Autodesk Inventor part; units mm, degrees
ref_plane "YZ Plane" through (0, 0, 0) normal (1, 0, 0) x (0, 1, 0)
ref_plane "XZ Plane" through (0, 0, 0) normal (0, 1, 0) x (-1, 0, 0)
ref_plane "XY Plane" through (0, 0, 0) normal (0, 0, 1) x (1, 0, 0)
sketch "スケッチ1" plane through (0, 0, 0) normal (0, 0, 1) x (1, 0, 0)
  circle A0 centre (12.3759, 55.251) radius 1.5
  circle A1 centre (22.7017, 77.6457) radius 1.5
  circle A2 centre (20.6799, 65) radius 1.5
  circle A3 centre (22.7017, 77.6457) radius 4.5
  circle A4 centre (20.6799, 65) radius 4.5
  circle A5 centre (12.3759, 55.251) radius 4.5
  line L0 (8.9502, 58.1689) -> (17.2542, 67.918)
  line L1 (18.2581, 78.3561) -> (16.2364, 65.7104)
  line L2 (27.1453, 76.9352) -> (25.1235, 64.2896)
  line L3 (15.8017, 52.333) -> (24.1057, 62.082)
  point P0 (0, 0)
  point P1 (0, 0)
  point P2 (16.4357, 66.957)
  dimension "d0" = 3
  dimension "d1" = 3
  dimension "d2" = 3
extrude "押し出し1" add sketch "スケッチ1" along normal blind 3
properties part number "段ばね抑え2" material "アセタール樹脂、白"
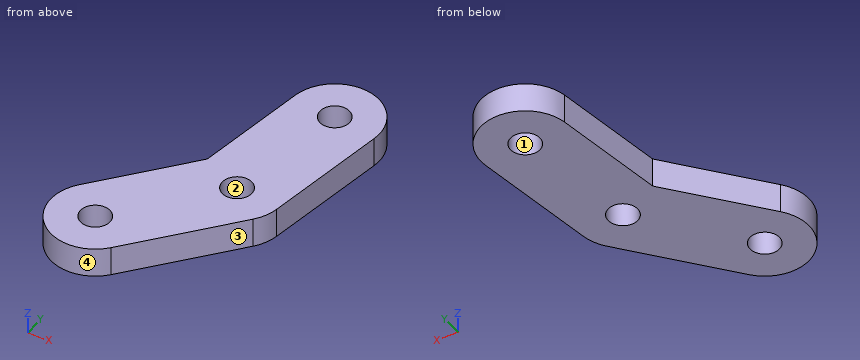
Here's how the part is built. I have some questions about the finished solid (model axes, mm). Face numbers are marked on the shaded views. Round coordinates to 2 decimals unless told otherwise and drop trailing zeros. Order: outer loops, then holes, each group sorted by start corner. A loop starts at its lowest first (then second) coordinate and runs counter-clockwise, first axis right, second up. Notation, with made-up numbers: (19, -32) -> (25, -32) arc R19 ccw to (25, -1) -> close; hole circle Ø1 at (25.5, -18). An arc over 180 degrees is marked (long way). Use CSV: the item, a comma, the result in double quotes.
1. I want a section at A-A on x = 12. List the corners of the cut face in (y, z) for me, and give its area (3 significant figures).
Recorded:
outline,"(50.77, 0) -> (53.8, 0) -> (53.8, 3) -> (50.77, 3) -> close; (56.7, 0) -> (61.75, 0) -> (61.75, 3) -> (56.7, 3) -> close"
area,"24.2 mm2"
2. Thinking about a two-plate mould opening in Y: for the marked faces 1, 2, 3 and 4, which applies, pulls with the +Y half, pulls with the -Y half, needs draft (parallel to the pull), parting line crosses it, or undercut?
Recorded:
face 1,"undercut"
face 2,"undercut"
face 3,"pulls with the -Y half"
face 4,"parting line crosses it"
3. I need wall thicknesses on line 1 along Y through (x, z) = (21.5, 0.85); line 2 along X through (y, z) = (79, 0.65); line 3 along Y through (x, z) = (11.75, 1.6). Which ranges of each line are inside material? Lowest first, please.
Recorded:
line 1,"y = 59.02 to 63.74, 66.26 to 76.75, 78.54 to 81.98"
line 2,"x = 18.41 to 22.06, 23.35 to 26.99"
line 3,"y = 50.79 to 53.89, 56.61 to 61.46"
4. I want a section at D-D on y = 79.5. List the corners of the cut face in (x, z) for me.
Recorded:
outline,"(18.6, 0) -> (26.8, 0) -> (26.8, 3) -> (18.6, 3) -> close"
5. I want a section at B-B on y = 56. List the corners of the cut face in (x, z) for me, and give its area (3 significant figures).
Recorded:
outline,"(7.94, 0) -> (11.08, 0) -> (11.08, 3) -> (7.94, 3) -> close; (13.68, 0) -> (18.93, 0) -> (18.93, 3) -> (13.68, 3) -> close"
area,"25.2 mm2"
6. I'm going to push a flat-ended pin straight in: P1, Ø1, axis at x = 16.5, z = 2, coming from the -Y side. Where does the tip first touch, or does it pass through?
Recorded:
P1,"stops at y = 52.57"
7. I want a section at C-C on z = 1.7. List the corners of the cut face in (x, y) for me, and give its area (3 significant figures).
Recorded:
outline,"(8.95, 58.17) arc R4.5 ccw to (15.8, 52.33) -> (24.11, 62.08) arc R4.5 ccw to (25.12, 64.29) -> (27.15, 76.94) arc R4.5 ccw to (18.26, 78.36) -> (16.44, 66.96) -> close; hole circle Ø3 at (12.38, 55.25); hole circle Ø3 at (20.68, 65); hole circle Ø3 at (22.7, 77.65)"
area,"273 mm2"
